The listing builds one solid part. Answer for the finished solid, in the listing's coordinates (mm). A direction names the side the tool comes from. Give positions to 0.01 mm unless a question says otherwise; leave off trailing zeros. Loops run counter-clockwise (first coordinate to the right, second up) from the corner with the lowest first, then second, coordinate; pieces in that order, holes last. Notation, with made-up numbers: M 35.5,-20 L 50.5,-20 A8 ccw 50.5,-9 Z; hole C 42,77.5 d3. An arc over 180 degrees is marked long. One line per item, written item: value. Start each with the question number.
Q1. Consider L1, parallel to X at y = -20, z = -0.9; L2, parallel to Z at x = 45, y = 17.5; L3, parallel to Z at x = 38.5, y = 13. Determine where each line is inside the solid, lowest interval first.
Q2. The mould has two halves that part along Z. Classify faces 1 (the flat face through (24.79, -36.94, -0.84)), 2 (the flat face through (46, -16, -1.7)), 3 (the flat face through (39, 15, -1.7)), 4 (the cylindrical face through (37.646, 19.188, 5.236)): +Z half, -Z half, draft (parallel to the pull), parting line (faces both ways), or undercut.
Q3. A cutting plane is placed at D-D, the plane y = 8. Determine the outline of the cut face in (x, z), and give its area (3 significant figures).
Q4. A cutting plane is placed at B-B, the plane x = 46.5. Determine the outline of the cut face in (y, z).
Q5. A cutting plane is placed at A-A, the plane y = -20. Determine the outline of the cut face in (x, z), and give its area (3 significant figures).
Q6. For faces 5 (the flat face through (35.969, 19.817, 8.013)), 6 (the flat face through (32.249, 24.024, 12.122)), 7 (the flat face through (33, -8, -1.7)), 8 (the flat face through (35, -20, -1.7)), 9 (the flat face through (35.26, 21.04, 6.6)), determine the directions among +Z, -Z, +X, -X, +Y, -Y from which every point of the face is accessible in a straight line to the end or side of a thin tool.
Q7. A cutting plane is placed at C-C, the plane z = 2. Determine the outline of the cut face in (x, y), and give its area (3 significant figures).
Q8. Flat-ended cylindrical pins translate along their axes: pin 1 (5 mm diameter, centred on x = 34, y = -19, fed in from +Z); pin 2 (17.5 mm diameter, centred on x = 35.5, y = 14, fed in from +Z); pin 3 (5 mm diameter, centred on x = 36.5, z = 0.5, fed in from +Y). Find the tip coordinate at first contact, or state that the pin passes through.
Autodesk Inventor part; units mm, degrees
ref_plane "Work Plane1" through (0, 0, -2) normal (0, 0, 1) x (1, 0, 0)
ref_plane "YZ Plane" through (0, 0, 0) normal (1, 0, 0) x (0, 1, 0)
ref_plane "XZ Plane" through (0, 0, 0) normal (0, 1, 0) x (-1, 0, 0)
sketch "Sketch1" plane through (0, 0, 0) normal (0, 0, 1) x (1, 0, 0)
  circle A0 centre (0, 0) radius 7.5
  line L0 (-21.2869, 0) -> (22.3896, 0) construction
  line L1 (0, 21.9302) -> (0, -69.0741) construction
  line L2 (24.9778, -67) -> (-24.9778, -67) construction
  line L3 (-17.5, -57) -> (17.5, -57)
  line L4 (17.5, -57) -> (17.5, -67)
  line L5 (17.5, -67) -> (-17.5, -67)
  line L6 (-17.5, -67) -> (-17.5, -57)
  line L7 (-37.5278, -67) -> (-18.5, -67)
  line L8 (-18.5, -67) -> (-18.5, -56)
  line L9 (-17.5, -62) -> (17.5, -62) construction
  line L10 (-18.5, -59) -> (-22.5, -59)
  line L11 (-22.5, -59) -> (-22.5, -65)
  line L12 (-22.5, -65) -> (-18.5, -65)
  line L13 (-18.5, -65) -> (-18.5, -59)
  line L14 (-17.5, -60) -> (-21.5, -60)
  line L15 (-21.5, -60) -> (-21.5, -64)
  line L16 (-21.5, -64) -> (-17.5, -64)
  line L17 (-17.5, -64) -> (-17.5, -60)
  line L18 (-18.5, -56) -> (-28.8675, -56)
  line L19 (17.5, -60) -> (21.5, -60)
  line L20 (21.5, -60) -> (21.5, -64)
  line L21 (21.5, -64) -> (17.5, -64)
  line L22 (17.5, -64) -> (17.5, -60)
  line L23 (18.5, -67) -> (18.5, -56)
  line L24 (18.5, -67) -> (37.5278, -67)
  line L25 (18.5, -65) -> (22.5, -65)
  line L26 (22.5, -65) -> (22.5, -59)
  line L27 (22.5, -59) -> (18.5, -59)
  line L28 (18.5, -59) -> (18.5, -65)
  line L29 (18.5, -56) -> (28.8675, -56)
  line L30 (-23.7704, -40) -> (28.6931, -40) construction
  line L31 (-17.1762, -35.75) -> (17.1762, -35.75)
  line L32 (-22.0836, -44.25) -> (22.0836, -44.25)
  circle A1 centre (0, -40) radius 2.25
  line L33 (-7.5, -16) -> (7.5, -16)
  line L34 (7.5, -16) -> (7.5, -21)
  line L35 (7.5, -26) -> (-7.5, -26)
  line L36 (-7.5, -26) -> (-7.5, -24)
  line L37 (7.5, -21) -> (-7.5, -21) construction
  line L38 (-7.5, -18) -> (-3.5, -18)
  line L39 (-3.5, -18) -> (-3.5, -21)
  line L40 (-3.5, -24) -> (-7.5, -24)
  line L41 (-7.5, -24) -> (-7.5, -23)
  line L42 (-8.5, -19) -> (-4.5, -19)
  line L43 (-4.5, -19) -> (-4.5, -23)
  line L44 (-4.5, -23) -> (-8.5, -23)
  line L45 (-8.5, -23) -> (-8.5, -19)
  line L46 (7.5, -18) -> (3.5, -18)
  line L47 (3.5, -18) -> (3.5, -21)
  line L48 (3.5, -24) -> (7.5, -24)
  line L49 (7.5, -24) -> (7.5, -18)
  line L50 (8.5, -19) -> (4.5, -19)
  line L51 (4.5, -19) -> (4.5, -23)
  line L52 (4.5, -23) -> (8.5, -23)
  line L53 (8.5, -23) -> (8.5, -19)
  line L54 (-9.815, -19) -> (-31.1769, -56)
  line L55 (-7.5056, -19) -> (-28.8675, -56)
  line L56 (7.5056, -19) -> (28.8675, -56)
  line L57 (-4.5, -21) -> (-8.5, -21)
  line L58 (4.5, -21) -> (8.5, -21)
  line L59 (-21.5, -62) -> (-17.5, -62)
  line L60 (17.5, -62) -> (21.5, -62)
  line L61 (-22.5, -62) -> (-18.5, -62)
  line L62 (22.5, -62) -> (18.5, -62)
  line L63 (-7.5, -21) -> (-3.5, -21)
  line L64 (3.5, -21) -> (7.5, -21)
  line L65 (-28.8675, -56) -> (-31.1769, -56)
  line L66 (28.8675, -56) -> (31.1769, -56)
  line L67 (-10.8853, -24.8539) -> (-12.6173, -23.8539)
  line L68 (10.8875, -24.8576) -> (12.6195, -23.8576)
  line L69 (7.5, -23) -> (7.5, -24)
  line L70 (-7.5, -23) -> (-7.5, -21)
  line L71 (-7.5, -24) -> (-7.5, -16)
  line L72 (7.5, -24) -> (7.5, -26)
  line L73 (-7.5, -21) -> (-7.5, -18)
  line L74 (-3.5, -21) -> (-3.5, -24)
  line L75 (3.5, -21) -> (3.5, -24)
  line L76 (7.5, -21) -> (7.5, -23)
  line L77 (-18.4752, 0) -> (-9.2376, 16)
  line L78 (-9.2376, 16) -> (9.2376, 16)
  line L79 (9.2376, 16) -> (18.4752, 0)
  line L80 (18.4752, 0) -> (9.2376, -16)
  line L81 (9.2376, -16) -> (-9.2376, -16)
  line L82 (-9.2376, -16) -> (-18.4752, 0)
  line L83 (-77.3649, 0) -> (-38.6825, 67) construction
  line L84 (-38.6825, 67) -> (38.6825, 67) construction
  line L85 (38.6825, 67) -> (77.3649, 0) construction
  line L86 (77.3649, 0) -> (38.6825, -67) construction
  line L87 (38.6825, -67) -> (-38.6825, -67) construction
  line L88 (-38.6825, -67) -> (-77.3649, 0) construction
  line L89 (-9.2376, -16) -> (-38.6825, -67) construction
  line L90 (9.2376, -16) -> (38.6825, -67) construction
  line L91 (0, -16.7974) -> (0, -26) construction
  line L92 (9.815, -19) -> (31.1769, -56)
  line L93 (-8.5, -19) -> (-9.815, -19)
  line L94 (8.5, -19) -> (9.815, -19)
  line L95 (-8.5, -23) -> (-9.815, -23)
  line L96 (8.5, -23) -> (9.815, -23)
  line L97 (-31.1769, -56) -> (-37.5278, -67)
  line L98 (31.1769, -56) -> (37.5278, -67)
  circle A2 centre (12.25, 0) radius 2.25
  circle A3 centre (6.125, 10.6088) radius 2.25
  circle A4 centre (-6.125, 10.6088) radius 2.25
  circle A5 centre (-12.25, 0) radius 2.25
  circle A6 centre (-6.125, -10.6088) radius 2.25
  circle A7 centre (6.125, -10.6088) radius 2.25
  line L99 (22.3723, -32.75) -> (39.5485, -3)
  line L100 (27.2798, -41.25) -> (49.3634, -3)
  circle A8 centre (34.641, -20) radius 2.25
  line L101 (39.5485, 3) -> (22.3723, 32.75)
  line L102 (49.3634, 3) -> (27.2798, 41.25)
  circle A9 centre (34.641, 20) radius 2.25
  line L103 (17.1762, 35.75) -> (-17.1762, 35.75)
  line L104 (22.0836, 44.25) -> (-22.0836, 44.25)
  circle A10 centre (0, 40) radius 2.25
  line L105 (-22.3723, 32.75) -> (-39.5485, 3)
  line L106 (-27.2798, 41.25) -> (-49.3634, 3)
  circle A11 centre (-34.641, 20) radius 2.25
  line L107 (-39.5485, -3) -> (-22.3723, -32.75)
  line L108 (-49.3634, -3) -> (-27.2798, -41.25)
  circle A12 centre (-34.641, -20) radius 2.25
  line L109 (22.3723, -32.75) -> (27.2798, -41.25)
  line L110 (49.3634, -3) -> (51.0955, 0)
  line L111 (49.3634, 3) -> (51.0955, 0)
  line L112 (39.5485, -3) -> (41.2805, 0)
  line L113 (39.5485, 3) -> (41.2805, 0)
  line L114 (7.3612, 4.25) -> (38.8268, 4.25)
  line L115 (7.3612, -4.25) -> (38.8268, -4.25)
  arc A13 (8.5, 0) -> (7.3612, 4.25) centre (0, 0) ccw
  arc A14 (7.3612, -4.25) -> (8.5, 0) centre (0, 0) ccw
  arc A15 (7.3612, 4.25) -> (7.3612, -4.25) centre (0, 0) ccw
  line L116 (22.3723, 32.75) -> (27.2798, 41.25)
  line L117 (35.5854, -9.8643) -> (42.9466, -14.1143)
  line L118 (42.9466, 14.1143) -> (35.5854, 9.8643)
  line L119 (26.3354, 25.8857) -> (33.6966, 30.1357)
  line L120 (26.3354, -25.8857) -> (33.6966, -30.1357)
  circle A16 centre (39.266, 11.9893) radius 10.9122
  circle A17 centre (39.266, -11.9893) radius 11.4144
  circle A18 centre (26.3354, -34.8015) radius 10.8288
  circle A19 centre (26.3354, 34.635) radius 11.4085
  point P0 (0, -57)
  point P1 (0, -67)
  point P2 (0, -62)
  point P3 (0, -21)
  dimension "d0" = 15
  dimension "d16" = 10
  dimension "d20" = 6
  dimension "d21" = 4
  dimension "d22" = 4
  dimension "d23" = 1
  dimension "d24" = 1
  dimension "d25" = 35
  dimension "d27" = 3
  dimension "d28" = 4
  dimension "d29" = 1
  dimension "d30" = 6
  dimension "d31" = 4
  dimension "d32" = 1
  dimension "d34" = 3
  dimension "d35" = 27
  dimension "d39" = 4.5
  dimension "d41" = 2
  dimension "d42" = 2
  dimension "d44" = 10
  dimension "d45" = 4
  dimension "d46" = 6
  dimension "d48" = 4
  dimension "d49" = 1
  dimension "d50" = 4
  dimension "d52" = 6
  dimension "d53" = 4
  dimension "d54" = 4
  dimension "d55" = 1
  dimension "d56" = 4
  dimension "d57" = 15
  dimension "d60" = 2
  dimension "d81" = 16
  dimension "d83" = 67
  dimension "d84" = 1
  dimension "d86" = 2
  dimension "d87" = 1
  dimension "d88" = 5
  dimension "d89" = 3
  dimension "d90" = 3
  dimension "d112" = 4.5
  dimension "d113" = 2.5
  dimension "d116" = 360
  dimension "d120" = 360
  dimension "d122" = 2
  dimension "d123" = 2
  dimension "d124" = 1
  dimension "d127" = 7
  dimension "d128" = 7
  dimension "d131" = 7
  dimension "d134" = 7
extrude "Extrusion8" add sketch "Sketch1" against normal blind 2 contours A18 L100 L120 L99 | L99 A17 A8 L100 A18 | L120 L100 L109 L99 | L99 L117 L100 A17 A8 | L99 L112 A17 L100 L117 | L112 L113 A16 L102 L111 L110 L100 A17 | L113 L101 L118 L102 A16 | A16 A9 L102 L118 L101 | L101 A19 L102 A16 A9 | L101 L119 L102 A19
bend part "Bend Part1" radius 1 angle 45 line through (42.9466, 14.1143, 0) along (-0.8660254, -0.5, 0) centre toward (0, 0, 1) moving side (-0.5, 0.8660254, 0) both sides no
ref_plane "Work Plane1" through (0, 0, -2) normal (0, 0, 1) x (1, 0, 0)
sketch "Sketch2" plane through (0, 0, -2) normal (0, 0, 1) x (1, 0, 0)
  circle A0 centre (26.3354, 34.635) radius 11.4085
  circle A1 centre (39.266, 11.9893) radius 10.9122
  circle A2 centre (39.266, -11.9893) radius 11.4144
  circle A3 centre (26.3354, -34.8015) radius 10.8288
  point P0 (0, 0)
extrude "Extrusion9" add sketch "Sketch2" along normal blind 0.3 contours A1 | A2 | A3
equation "\"d20\" = hinge_w"
equation "\"d21\" = hinge_d"
equation "\"d22\" = hinge_w - 2 * hinge_sp"
equation "\"d23\" = hinge_sp"
equation "\"d24\" = sp"
equation "\"d28\" = hinge_w - 2 * hinge_sp"
equation "\"d29\" = sp"
equation "\"d30\" = hinge_w"
equation "\"d31\" = hinge_d"
equation "\"d32\" = hinge_sp"
equation "\"d39\" = screw"
equation "\"d45\" = hinge_d"
equation "\"d46\" = hinge_w"
equation "\"d48\" = hinge_d"
equation "\"d49\" = hinge_sp"
equation "\"d50\" = hinge_w - 2 * hinge_sp"
equation "\"screw\" = 4.5"
equation "\"k\" = 0.4"
equation "\"sp\" = 1"
equation "\"d14\" = sp"
equation "\"d15\" = sp"
equation "\"d19\" = sp"
equation "\"hinge_d\" = 4"
equation "\"hinge_w\" = 6"
equation "\"hinge_sp\" = 1"
properties part number "RobotBase" material "Glass"
Answer block:
1. L1: 29.73 to 32.39, 36.89 to 39.55
1. L2: -2 to -1.7
1. L3: -2 to 0.84
2. face 1: draft
2. face 2: +Z half
2. face 3: undercut
2. face 4: undercut
3. outline: M 29.11,-2 L 49.42,-2 L 49.42,-1.7 L 46.48,-1.7 L 46.48,0 L 36.66,0 L 36.66,-1.7 L 29.11,-1.7 Z
3. area: 22.8 mm^2
4. outline: M -20.82,-2 L 20.16,-2 L 20.16,-1.7 L 7.96,-1.7 L 7.96,0 L -7.96,0 L -7.96,-1.7 L -20.82,-1.7 Z
5. outline: M 29.73,-2 L 47.4,-2 L 47.4,-1.7 L 39.55,-1.7 L 39.55,0 L 36.89,0 L 36.89,-1.7 L 32.39,-1.7 L 32.39,0 L 29.73,0 Z
5. area: 14.3 mm^2
6. face 5: +Z, +X, -Y
6. face 6: +Z, -X, +Y
6. face 7: +Z, -X
6. face 8: +Z
6. face 9: -X, +Y
7. outline: M 32.96,14.4 L 34.38,11.96 L 41.74,16.21 L 40.33,18.65 Z
7. area: 24.0 mm^2
8. pin 1: z = 0
8. pin 2: z = 11.96
8. pin 3: y = 22.79
